```python
from build123d import *

# Parameters (mm, degrees)
EXTRUDE_1_DEPTH      = 3.9
EXTRUDE_1_DEPTH_BACK = 7.5
SKETCH_1_R           = 5
SKETCH_1_R_2         = 3
CHAMFER_1_SIZE       = 0.5
SKETCH_2_W           = 1.242269364
SKETCH_2_H           = 0.9
EXTRUDE_1_2_DEPTH    = 3


with BuildPart() as part:
    # 草图1 → Extrude 1 (new, two sides: drawn at the far end of the back side and taken through both)
    with BuildSketch(Plane.XY.offset(-EXTRUDE_1_DEPTH_BACK)):
        Circle(SKETCH_1_R)
        Circle(SKETCH_1_R_2, mode=Mode.SUBTRACT)
    extrude(amount=EXTRUDE_1_DEPTH + EXTRUDE_1_DEPTH_BACK)

    # 倒角1
    chamfer_1_edges = [part.edges().sort_by_distance(p)[0] for p in [
        (-3, 0, -7.5),
        (-3, 0, 3.9),
    ]]
    chamfer(chamfer_1_edges, length=CHAMFER_1_SIZE)

    # 草图2 → Extrude 1 2 (add)
    with BuildSketch(Plane.XY):
        with Locations((-2.68480736, 0)):
            Rectangle(SKETCH_2_W, SKETCH_2_H)
        with Locations((2.68480736, 0)):
            Rectangle(SKETCH_2_W, SKETCH_2_H)
    extrude(amount=EXTRUDE_1_2_DEPTH)


solid = part.part
```
Geometry check sheet. Reference: the model listing, model coordinates, mm. A direction names the side the tool comes from. Round coordinates to 2 decimals unless told otherwise and drop trailing zeros. Write each loop counter-clockwise with the first axis right and the second up, starting at its lowest first coordinate (ties: lowest second). Pieces come first, ordered by that corner, then holes. Notation, with made-up numbers: (-16, 23.25) -> (-12, 23.25) arc R24 cw to (-12, 48.25) -> close; hole circle Ø4 at (47, 70.25). An arc over 180 degrees is marked (long way). Put each result on its own line as item: value.
1) Thickness scan on probe 1 along Y at (x, z) = (0, -0.5); probe 2 along Y at (x, z) = (-1, 0.75); probe 3 along X at (y, z) = (-0.5, -4.75). Record the ranges inside material, lowest first. Write a range as from..to.
Recorded:
probe 1: y = -5..-3, 3..5
probe 2: y = -4.9..-2.83, 2.83..4.9
probe 3: x = -4.97..-2.96, 2.96..4.97
2) Cross-section at A-A, the plane x = 0. Enter the section's corners in (y, z).
Recorded:
outline: (-5, -7.5) -> (-3.5, -7.5) -> (-3, -7) -> (-3, 3.4) -> (-3.5, 3.9) -> (-5, 3.9) -> close; (3, -7) -> (3.5, -7.5) -> (5, -7.5) -> (5, 3.9) -> (3.5, 3.9) -> (3, 3.4) -> close
3) Release check for a two-part mould opening along Y. For faces 1 (the face through (2.2, -3.3, 3.9)), 2 (the face through (-2.064, 0, 1)), 3 (the face through (-1.08, -4.88, -1.88)) record: pulls with the +Y half, pulls with the -Y half, needs draft (parallel to the pull), parting line crosses it, or undercut.
Recorded:
face 1: needs draft
face 2: undercut
face 3: parting line crosses it
4) Depth check by flat-ended pin: P1, Ø3, axis at x = 3.5, z = -3, coming from the +Y side; P2, Ø0.7, axis at x = 2.5, y = 0, coming from the +Z side; P3, Ø1, axis at x = 2.5, z = 1, coming from the -Y side. Enter the tip coordinate at first touch or a pass-through.
Recorded:
P1: stops at y = 4.58
P2: stops at z = 3
P3: stops at y = -4.58
5) Cross-section at B-B, the plane y = 0. Enter the section's corners in (x, z).
Recorded:
outline: (-5, -7.5) -> (-3.5, -7.5) -> (-3, -7) -> (-3, 0) -> (-2.06, 0) -> (-2.06, 3) -> (-3, 3) -> (-3, 3.4) -> (-3.5, 3.9) -> (-5, 3.9) -> close; (2.06, 0) -> (3, 0) -> (3, -7) -> (3.5, -7.5) -> (5, -7.5) -> (5, 3.9) -> (3.5, 3.9) -> (3, 3.4) -> (3, 3) -> (2.06, 3) -> close
6) Cross-section at C-C, the plane z = 1.25. Enter the section's corners in (x, y), plus the area to 3 significant figures.
Recorded:
outline: circle Ø10 at (0, 0); hole (-2.97, -0.45) arc R3 ccw to (2.97, -0.45) -> (2.06, -0.45) -> (2.06, 0.45) -> (2.97, 0.45) arc R3 ccw to (-2.97, 0.45) -> (-2.06, 0.45) -> (-2.06, -0.45) -> close
area: 51.9 mm2
7) Access from +Z, -Z, +X, -X, +Y, -Y to the whole of each face (thin tool, end or side, straight path). Record for faces 4 (the face through (2.5, 0.45, 1.5)), 5 (the face through (-2.5, 0, 0)), 6 (the face through (-2.5, 0, 3)).
Recorded:
face 4: +Z, -Z
face 5: -Z
face 6: +Z
8) Cross-section at D-D, the plane z = -2.5. Enter the section's corners in (x, y), plus the area to 3 significant figures.
Recorded:
outline: circle Ø10 at (0, 0); hole circle Ø6 at (0, 0)
area: 50.3 mm2
